Source: CAD feature listing. Evaluate the final solid. Frame: model axes, mm. A direction names the side the tool comes from. Give positions to 0.01 mm unless a question says otherwise; leave off trailing zeros. Write each loop counter-clockwise with the first axis right and the second up, starting at its lowest first coordinate (ties: lowest second). Pieces come first, ordered by that corner, then holes.
```python
from build123d import *

# Parameters (mm, degrees)
EXTRUDE_1_DEPTH      = 20
EXTRUDE_1_DEPTH_BACK = 20
EXTRUDE_2_DEPTH      = 15
EXTRUDE_2_DEPTH_BACK = 15
CHAMFER_1_SIZE       = 1
HOLE_WIZARD_5_0_1_D  = 5
FILLET_1_R           = 0.2


with BuildPart() as part:
    # Эскиз1 → Бобышка-Вытянуть1 (new, two sides: drawn at the far end of the back side and taken through both)
    with BuildSketch(Plane.XY.offset(-EXTRUDE_1_DEPTH_BACK)):
        with BuildLine():
            Line((17.5, -12.5), (-17.5, -12.5))
            ThreePointArc((-17.5, -12.5), (-26.338834764831844, -8.838834764831844), (-30.000000000000004, 0))
            Line((-30.000000000000004, 0), (-25, 0))
            ThreePointArc((-25, 0), (-17.5, -7.499999999999998), (-10.000000000000002, 0))
            Line((-10.000000000000002, 0), (10.000000000000002, 0))
            ThreePointArc((10.000000000000002, 0), (17.5, -7.499999999999998), (25, 0))
            Line((25, 0), (30.000000000000004, 0))
            ThreePointArc((30.000000000000004, 0), (26.338834764831844, -8.838834764831843), (17.5, -12.5))
        make_face()
    extrude(amount=EXTRUDE_1_DEPTH + EXTRUDE_1_DEPTH_BACK)

    # Эскиз2 → Бобышка-Вытянуть2 (add, two sides: drawn at the far end of the back side and taken through both)
    with BuildSketch(Plane.XY.offset(-EXTRUDE_2_DEPTH_BACK)):
        with BuildLine():
            Line((30.000000000000004, 0), (35, 0))
            Line((35, 0), (35, -12.499999999999996))
            Line((35, -12.499999999999996), (17.5, -12.5))
            Line((17.5, -12.5), (-17.500000000000004, -12.5))
            Line((-17.500000000000004, -12.5), (-35, -12.499999999999996))
            Line((-35, -12.499999999999996), (-35, 0))
            Line((-35, 0), (-30.000000000000004, 1.53e-15))
            Line((-30.000000000000004, 1.53e-15), (-25, 9.2e-16))
            ThreePointArc((-25, 9.2e-16), (-17.5, -7.499999999999998), (-10.000000000000002, 0))
            Line((-10.000000000000002, 0), (10.000000000000002, 9.2e-16))
            ThreePointArc((10.000000000000002, 9.2e-16), (17.5, -7.499999999999998), (25, 0))
            Line((25, 0), (30.000000000000004, 0))
        make_face()
    extrude(amount=EXTRUDE_2_DEPTH + EXTRUDE_2_DEPTH_BACK)

    # Фаска1
    chamfer_1_edges = [part.edges().sort_by_distance(p)[0] for p in [
        (35, -12.499999999999996, 0),
        (-35, -12.499999999999996, 0),
    ]]
    chamfer(chamfer_1_edges, length=CHAMFER_1_SIZE)

    # Отверстия под штифты Ø5.0 мм1 (through all)
    with Locations(Plane(origin=(0, 0, 0), x_dir=(1, 0, 0), z_dir=(0, 1, 0))):
        with Locations((0, 15), (0, -15), (-30, -7.5), (-30, 7.5), (30, 7.5), (30, -7.5)):
            Hole(HOLE_WIZARD_5_0_1_D / 2)

    # Скругление1
    # the kernel refuses this fillet: 0.2 mm, written as the material it adds along each edge
    with BuildSketch(Plane(origin=(-17.5, 4.44e-15, -15), x_dir=(0.19874807030113847, -0.9800506132601386, 0), z_dir=(0.9800506132601386, 0.19874807030113847, 0))) as fillet_1_piece_1_section:
        with BuildLine():
            CenterArc((12.500000000000004 + FILLET_1_R, FILLET_1_R), FILLET_1_R, 180, 90)
            Line((12.500000000000004, FILLET_1_R), (12.500000000000004, 0))
            Line((12.500000000000004, 0), (12.500000000000004 + FILLET_1_R, 0))
        make_face()
    fillet_1_piece_1 = revolve(axis=Axis((-17.5, 4.44e-15, -15), (0, 0, -1)), revolution_arc=101.46375913899153, mode=Mode.PRIVATE)
    fillet_1_piece_1 = split(fillet_1_piece_1, bisect_by=Plane(origin=(-17.5, -12.5, -15), z_dir=(0, 1, 0)), keep=Keep.TOP, mode=Mode.PRIVATE)
    add(fillet_1_piece_1)
    with BuildSketch(Plane(origin=(-17.5, 4.44e-15, 15), x_dir=(0.19874807030113847, -0.9800506132601386, 0), z_dir=(0.9800506132601386, 0.19874807030113847, 0))) as fillet_1_piece_2_section:
        with BuildLine():
            CenterArc((12.500000000000004 + FILLET_1_R, -FILLET_1_R), FILLET_1_R, 90, 90)
            Line((12.500000000000004, -FILLET_1_R), (12.500000000000004, 0))
            Line((12.500000000000004, 0), (12.500000000000004 + FILLET_1_R, 0))
        make_face()
    fillet_1_piece_2 = revolve(axis=Axis((-17.5, 4.44e-15, 15), (0, 0, -1)), revolution_arc=101.46375913899153, mode=Mode.PRIVATE)
    fillet_1_piece_2 = split(fillet_1_piece_2, bisect_by=Plane(origin=(-17.5, -12.5, 15), z_dir=(0, 1, 0)), keep=Keep.TOP, mode=Mode.PRIVATE)
    add(fillet_1_piece_2)
    with BuildSketch(Plane(origin=(17.499999999999993, 1.199e-14, 15), x_dir=(1, -9.6e-16, 0), z_dir=(9.6e-16, 1, 0))) as fillet_1_piece_3_section:
        with BuildLine():
            CenterArc((12.50000000000001 + FILLET_1_R, -FILLET_1_R), FILLET_1_R, 90, 90)
            Line((12.50000000000001 + FILLET_1_R, 0), (12.50000000000001, 0))
            Line((12.50000000000001, 0), (12.50000000000001, -FILLET_1_R))
        make_face()
    fillet_1_piece_3 = revolve(axis=Axis((17.499999999999993, 1.199e-14, 15), (0, 0, -1)), revolution_arc=101.46375913899143, mode=Mode.PRIVATE)
    fillet_1_piece_3 = split(fillet_1_piece_3, bisect_by=Plane(origin=(17.499999999999993, -12.5, 15), z_dir=(0, 1, 0)), keep=Keep.TOP, mode=Mode.PRIVATE)
    add(fillet_1_piece_3)
    with BuildSketch(Plane(origin=(17.499999999999993, 1.199e-14, -15), x_dir=(1, -9.6e-16, 0), z_dir=(9.6e-16, 1, 0))) as fillet_1_piece_4_section:
        with BuildLine():
            CenterArc((12.50000000000001 + FILLET_1_R, FILLET_1_R), FILLET_1_R, 180, 90)
            Line((12.50000000000001 + FILLET_1_R, 0), (12.50000000000001, 0))
            Line((12.50000000000001, 0), (12.50000000000001, FILLET_1_R))
        make_face()
    fillet_1_piece_4 = revolve(axis=Axis((17.499999999999993, 1.199e-14, -15), (0, 0, -1)), revolution_arc=101.46375913899143, mode=Mode.PRIVATE)
    fillet_1_piece_4 = split(fillet_1_piece_4, bisect_by=Plane(origin=(17.499999999999993, -12.5, -15), z_dir=(0, 1, 0)), keep=Keep.TOP, mode=Mode.PRIVATE)
    add(fillet_1_piece_4)


solid = part.part
```
1. Section query B-B (z = -3.5). Return loops of the section in (x, y).
2. Pull-direction query (Z, two-part tool) for faces 1 (the cylindrical face through (32.5, -6.3, 7.4)), 2 (the cylindrical face through (-26.241, -8.935, 17.566)), 3 (the flat face through (-31, -8, -15)), 4 (the flat face through (0, -6, 20)); classes: pulls with the +Z half, pulls with the -Z half, needs draft (parallel to the pull), parting line crosses it, or undercut.
3. Section query D-D (y = -4.25). Give the number of separate pieces and of enclosed holes in the cut face, plus the area to 3 significant figures.
4. Section query A-A (z = 7.5). Return loops of the section in (x, y), plus the area to 3 significant figures.
5. Access query for faces 5 (the cylindrical face through (0.54, -6.34, -12.56)), 6 (the flat face through (31, -8, 15)), 7 (the cylindrical face through (26.435, -8.741, -17.634)). Directions: +Z, -Z, +X, -X, +Y, -Y. A direction counts if a zero-diameter tool reaches every point of the face in a straight line with its end or side. Return the directions, or none.
6. Line query: probe 1 along Z at (x, y) = (-30, -8.25); probe 2 along X at (y, z) = (-4.25, -10.5); probe 3 along X at (y, z) = (-6, 9.5). Output: solid intervals per line, ascending.
7. Pin query (flat end, axial travel): P1, Ø4, axis at x = -30, z = -7.5, coming from the +Y side; P2, Ø6, axis at y = -5.5, z = -16, coming from the -X side; P3, Ø4, axis at x = -30, y = -9, coming from the -Z side. Return the tip coordinate at first contact, or that it passes through.
8. Section query C-C (x = 13). Return loops of the section in (y, z).
The answers:
1. outline: (-35, -11.5) - (-34, -12.5) - (34, -12.5) - (35, -11.5) - (35, 0) - (25, 0) arc R7.5 cw to (10, 0) - (-10, 0) arc R7.5 cw to (-25, 0) - (-35, 0) - close
2. face 1: undercut
2. face 2: needs draft
2. face 3: pulls with the -Z half
2. face 4: pulls with the +Z half
3. separate pieces: 3
3. enclosed holes: 6
3. area: 1,580 mm2
4. outline: (-35, -11.5) - (-34, -12.5) - (-32.5, -12.5) - (-32.5, 0) - (-35, 0) - close; (-27.5, -12.5) - (27.5, -12.5) - (27.5, 0) - (25, 0) arc R7.5 cw to (10, 0) - (-10, 0) arc R7.5 cw to (-25, 0) - (-27.5, 0) - close; (32.5, -12.5) - (34, -12.5) - (35, -11.5) - (35, 0) - (32.5, 0) - close
4. area: 572 mm2
5. face 5: +Y, -Y
5. face 6: +Z, +X, -Y
5. face 7: -Z, +X, -Y
6. probe 1: z = -15 to -10, -5 to 5, 10 to 15
6. probe 2: x = -35 to -23.68, -11.32 to 11.32, 23.68 to 35
6. probe 3: x = -35 to -31.5, -28.5 to -22, -13 to 13, 22 to 28.5, 31.5 to 35
7. P1: passes through
7. P2: stops at x = -35
7. P3: stops at z = -15
8. outline: (-12.5, -20) - (-6, -20) - (-6, 20) - (-12.5, 20) - close
